from build123d import *

# Parameters (mm, degrees)
SKETCH1_R           = 31
SKETCH1_R_2         = 28
BOSS_EXTRUDE1_DEPTH = 30
BOSS_EXTRUDE2_START = -10
BOSS_EXTRUDE2_DEPTH = 10
CUT_EXTRUDE1_DEPTH  = 51
SKETCH4_W           = 5
SKETCH4_H           = 10
SKETCH4_R           = 1.25
BOSS_EXTRUDE3_DEPTH = 2
SKETCH4_3_W         = 10
SKETCH4_3_H         = 2
BOSS_EXTRUDE4_DEPTH = 1
CUT_EXTRUDE2_START  = -6
SKETCH4_4_R         = 1.25
CUT_EXTRUDE2_DEPTH  = 6
FILLET1_R           = 1
FILLET3_R           = 11


with BuildPart() as part:
    # Sketch1 → Boss-Extrude1 (new body)
    with BuildSketch(Plane(origin=(0, 0, 0), x_dir=(1, 0, 0), z_dir=(0, 1, 0))):
        with Locations(Location((0, 0, 0), (0, 0, 270))):
            Circle(SKETCH1_R)
        with Locations(Location((0, 0, 0), (0, 0, 270))):
            Circle(SKETCH1_R_2, mode=Mode.SUBTRACT)
    extrude(amount=-BOSS_EXTRUDE1_DEPTH)

    # Sketch2 → Boss-Extrude2 (add)
    with BuildSketch(Plane.XZ.offset(30).offset(BOSS_EXTRUDE2_START)):
        with BuildLine():
            Line((-24.701905706, -13.183924092), (24.701905706, -13.183924092))
            ThreePointArc((24.701905706, -13.183924092), (0, -28), (-24.701905706, -13.183924092))
        make_face()
    extrude(amount=BOSS_EXTRUDE2_DEPTH)

    # Sketch3 → Cut-Extrude1 (cut)
    with BuildSketch(Plane.XY.offset(-13.183924092)):
        with BuildLine():
            Line((-10, -30), (10, -30))
            ThreePointArc((10, -30), (0, -20), (-10, -30))
        make_face()
    extrude(amount=CUT_EXTRUDE1_DEPTH, mode=Mode.SUBTRACT)

    # Sketch4 → Boss-Extrude3 (add)
    # profile 1 of 2: a face of its own
    with BuildSketch(Plane.XY.offset(-13.183924092)):
        with Locations((-7.5, -25)):
            Rectangle(SKETCH4_W, SKETCH4_H)
        with Locations((-7.5, -25)):
            Circle(SKETCH4_R, mode=Mode.SUBTRACT)
    # profile 2 of 2: a face of its own
    with BuildSketch(Plane.XY.offset(-13.183924092)):
        with Locations((7.5, -25)):
            Rectangle(SKETCH4_W, SKETCH4_H)
        with Locations((7.5, -25)):
            Circle(SKETCH4_R, mode=Mode.SUBTRACT)
    extrude(amount=BOSS_EXTRUDE3_DEPTH)

    # Sketch4<3> → Boss-Extrude4 (add)
    with BuildSketch(Plane.XY.offset(-13.183924092)):
        with Locations((0, -25)):
            Rectangle(SKETCH4_3_W, SKETCH4_3_H)
    extrude(amount=BOSS_EXTRUDE4_DEPTH)

    # Sketch4<4> → Cut-Extrude2 (cut)
    with BuildSketch(Plane.XY.offset(-13.183924092).offset(CUT_EXTRUDE2_START)):
        with Locations((-7.5, -25)):
            Circle(SKETCH4_4_R)
        with Locations((7.5, -25)):
            Circle(SKETCH4_4_R)
    extrude(amount=CUT_EXTRUDE2_DEPTH, mode=Mode.SUBTRACT)

    # Fillet1
    fillet1_edges = [part.edges().sort_by_distance(p)[0] for p in [
        (0, -24, -12.183924092),
        (0, -26, -12.183924092),
    ]]
    fillet(fillet1_edges, radius=FILLET1_R - 0.0001)  # a hair under: the kernel refuses the full size

    # Chamfer1: read off the stored shape, not the designer's step
    # Chamfer1 outline → Chamfer1 (revolve, cut)
    with BuildSketch(Plane.XY):
        Polygon((31, -15.699333743), (30, -30), (31, -30), align=None)
    revolve(axis=Axis((0, 0, 0), (0, 1, 0)), mode=Mode.SUBTRACT)

    # Fillet3
    fillet3_edges = [part.edges().sort_by_distance(p)[0] for p in [
        (0, -20, -28),
    ]]
    fillet(fillet3_edges, radius=FILLET3_R)


solid = part.part
Here's how the part is built. I have some questions about the finished solid (model axes, mm). A direction names the side the tool comes from. Coordinates: 2 decimals unless noted, no trailing zeros. Loops run counter-clockwise (first coordinate to the right, second up) from the corner with the lowest first, then second, coordinate; pieces in that order, holes last.
1. For P1, Ø3, axis at x = 7.5, y = -25, coming from the +Z side; P2, Ø1.2, axis at x = -7.5, y = -25, coming from the +Z side; P3, Ø3, axis at x = -7.5, y = -25, coming from the -Z side, each with a flat end and sliding along its axis, tell me the tip position at first contact or that it passes through.
2. Imagine slicing it at D-D, the plane y = -16.5. Please give me the cut outline in (x, z).
3. If we mould it in two halves opening along Y, with no side actions, what happens to faces 5 (the cylindrical face through (6.25, -24.95, -15.24)), 6 (the flat face through (-27.4, 0, -7)), 7 (the flat face through (-19, -24, -13.184))? For each: pulls with the +Y half, pulls with the -Y half, needs draft (parallel to the pull), parting line crosses it, or undercut.
4. For faces 1 (the conical face through (-3.955, -24.539, -30.123)), 2 (the flat face through (10, -25, -12)), 3 (the flat face through (0, -28, -13.184)), 4 (the flat face through (0, -20, -14)), which set-ups out of +Z, -Z, +X, -X, +Y, -Y let a thin tool reach every point of the face, with its end or its side?
5. Imagine slicing it at B-B, the plane y = -11. Please give me the cut outline in (x, z).
6. I need wall thicknesses on L1, parallel to Y at x = 7.5, z = -13.25; L2, parallel to X at y = -19, z = 14.5; L3, parallel to X at y = -11, z = -7. Which ranges of each line are inside material? Lowest first, please.
7. Imagine slicing it at C-C, the plane y = -6. Please give me the cut outline in (x, z).
8. Imagine slicing it at A-A, the plane z = 0. Please give me the cut outline in (x, y), and give its area (3 significant figures).
Taken from the geometry:
1. P1: stops at z = 29.49
1. P2: stops at z = -19.18
1. P3: stops at z = -29.77
2. outline: circle Ø61.89 at (0, 0); hole (-24.7, -13.18) - (-21.3, -13.18) arc R25.05 ccw to (21.3, -13.18) - (24.7, -13.18) arc R28 ccw (long way) to start
3. face 5: undercut
3. face 6: pulls with the +Y half
3. face 7: needs draft
4. face 1: -Y
4. face 2: +Y, -Y
4. face 3: +Z, -Y
4. face 4: +Y
5. outline: circle Ø62 at (0, 0); hole (-24.7, -13.18) - (-24.49, -13.18) arc R27.82 ccw to (24.49, -13.18) - (24.7, -13.18) arc R28 ccw (long way) to start
6. L1: y = -30 to -26.25, -23.75 to -20
6. L2: x = -27.14 to -23.95, 23.95 to 27.14
6. L3: x = -30.2 to -27.11, 27.11 to 30.2
7. outline: circle Ø62 at (0, 0); hole circle Ø56 at (0, 0)
8. outline: (-31, -15.7) - (-30, -30) - (-28, -30) - (-28, 0) - (-31, 0) - close; (28, -30) - (30, -30) - (31, -15.7) - (31, 0) - (28, 0) - close
8. area: 166 mm2
